```python
from build123d import *

# Parameters (mm, degrees)
F2_DEPTH = 6
F1_W     = 24.3
F1_H     = 10.5
F1_R     = 2.5
F1_W_2   = 4.5
F1_H_2   = 3.75
F1_R_2   = 1.5
F1_R_3   = 20
F3_DEPTH = 6.001
F4_R     = 1
F5_R     = 0.5
F6_R     = 4
F7_R     = 5
F8_R     = 10


# Not quite as in the source:
# - a feature names something its author has since deleted; it is built from what else it names


with BuildPart() as f2:
    # F0 (on Top) → F2 (new body)
    with BuildSketch(Plane.XY):
        with BuildLine():
            Line((-38.5, 52.75), (-38.5, 41.5))
            Line((-38.5, 41.5), (-38.5, -23.99190475))
            ThreePointArc((-38.5, -23.99190475), (-34.7157474887, -63.5877422109), (-23.5, -101.75))
            Line((-23.5, -101.75), (23.5, -101.75))
            ThreePointArc((23.5, -101.75), (34.7157474887, -63.5877422109), (38.5, -23.99190475))
            Line((38.5, -23.99190475), (38.5, 41.5))
            Line((38.5, 41.5), (38.5, 52.75))
            Line((38.5, 52.75), (-38.5, 52.75))
        make_face()
    extrude(amount=F2_DEPTH)

    # F1 (on Top) → F3 (cut, through all)
    with BuildSketch(Plane.XY):
        with Locations((0, -41.5)):
            Rectangle(F1_W, F1_H)
        with BuildLine():
            ThreePointArc((-2.25, -33.25), (-3, -34), (-2.25, -34.75))
            Line((-2.25, -34.75), (2.25, -34.75))
            ThreePointArc((2.25, -34.75), (3, -34), (2.25, -33.25))
            Line((2.25, -33.25), (-2.25, -33.25))
        make_face()
        with BuildLine():
            ThreePointArc((-21, -21.25), (-18.4168483179, -27.5611508459), (-12.15, -30.25))
            Line((-12.15, -30.25), (12.15, -30.25))
            ThreePointArc((12.15, -30.25), (18.4168483179, -27.5611508459), (21, -21.25))
            ThreePointArc((21, -21.25), (25.387505004, -8.75), (21, 3.75))
            Line((21, 3.75), (-21, 3.75))
            ThreePointArc((-21, 3.75), (-25.387505004, -8.75), (-21, -21.25))
        make_face()
        with Locations((-30, 7.75)):
            Circle(F1_R)
        with Locations((-30, 27.75)):
            Circle(F1_R)
        with Locations((30, 7.75)):
            Circle(F1_R)
        with Locations((30, 27.75)):
            Circle(F1_R)
        with Locations((20.35, 41.5)):
            Rectangle(F1_W, F1_H)
        with BuildLine():
            ThreePointArc((18.1, 34.75), (17.35, 34), (18.1, 33.25))
            Line((18.1, 33.25), (22.6, 33.25))
            ThreePointArc((22.6, 33.25), (23.35, 34), (22.6, 34.75))
            Line((22.6, 34.75), (18.1, 34.75))
        make_face()
        with BuildLine():
            ThreePointArc((-22.6, 34.75), (-23.35, 34), (-22.6, 33.25))
            Line((-22.6, 33.25), (-18.1, 33.25))
            ThreePointArc((-18.1, 33.25), (-17.35, 34), (-18.1, 34.75))
            Line((-18.1, 34.75), (-22.6, 34.75))
        make_face()
        with Locations((-20.35, 41.5)):
            Rectangle(F1_W, F1_H)
        with Locations((-20.35, 50.875)):
            Rectangle(F1_W_2, F1_H_2)
        with Locations((20.35, 50.875)):
            Rectangle(F1_W_2, F1_H_2)
        with Locations((0, 46.75)):
            Circle(F1_R_2)
        with Locations((30, -4.25)):
            Circle(F1_R_2)
        with Locations((-30, -4.25)):
            Circle(F1_R_2)
        with Locations((0, -75.75)):
            Circle(F1_R_3)
        with BuildLine():
            ThreePointArc((-2.25, -48.25), (-3, -49), (-2.25, -49.75))
            Line((-2.25, -49.75), (2.25, -49.75))
            ThreePointArc((2.25, -49.75), (3, -49), (2.25, -48.25))
            Line((2.25, -48.25), (-2.25, -48.25))
        make_face()
        with Locations((16, -59.75)):
            Circle(F1_R_2)
        with Locations((-16, -59.75)):
            Circle(F1_R_2)
        with Locations((16, -91.75)):
            Circle(F1_R_2)
        with Locations((-16, -91.75)):
            Circle(F1_R_2)
    extrude(amount=F3_DEPTH, mode=Mode.SUBTRACT)

    # F4
    f4_edges = [f2.edges().sort_by_distance(p)[0] for p in [
        (12.15, -36.25, 3),
        (-12.15, -36.25, 3),
        (-12.15, -46.75, 3),
        (12.15, -46.75, 3),
        (8.2, 46.75, 3),
        (-32.5, 46.75, 3),
        (-32.5, 36.25, 3),
        (-8.2, 46.75, 3),
        (-8.2, 36.25, 3),
        (32.5, 36.25, 3),
        (8.2, 36.25, 3),
        (32.5, 46.75, 3),
    ]]
    fillet(f4_edges, radius=F4_R)

    # F5
    f5_edges = [f2.edges().sort_by_distance(p)[0] for p in [
        (18.1, 49, 3),
        (22.6, 49, 3),
        (-18.1, 49, 3),
        (-22.6, 49, 3),
        (-22.6, 52.75, 3),
        (-18.1, 52.75, 3),
        (18.1, 52.75, 3),
        (22.6, 52.75, 3),
    ]]
    fillet(f5_edges, radius=F5_R)

    # F6
    f6_edges = [f2.edges().sort_by_distance(p)[0] for p in [
        (-21, 3.75, 3),
        (21, 3.75, 3),
    ]]
    fillet(f6_edges, radius=F6_R)

    # F7
    f7_edges = [f2.edges().sort_by_distance(p)[0] for p in [
        (-23.5, -101.75, 3),
        (23.5, -101.75, 3),
        (-38.5, 52.75, 3),
        (38.5, 52.75, 3),
    ]]
    fillet(f7_edges, radius=F7_R)

    # F8
    f8_edges = [f2.edges().sort_by_distance(p)[0] for p in [
        (-21, -21.25, 3),
        (21, -21.25, 3),
    ]]
    fillet(f8_edges, radius=F8_R)


solid = f2.part
```
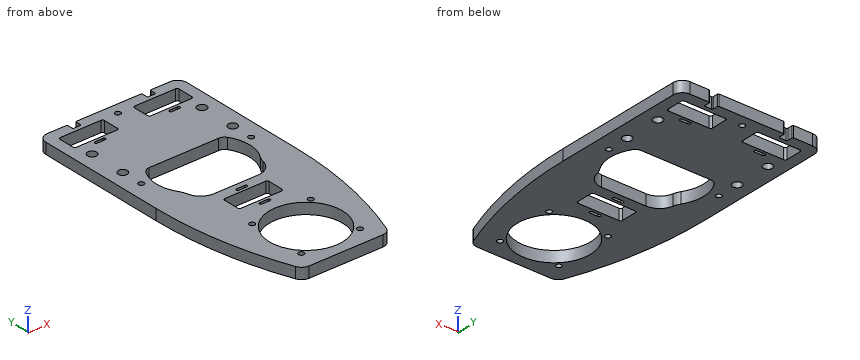
CAD build for the part. Positions are in the model's coordinates, mm. Round coordinates to 2 decimals unless told otherwise and drop trailing zeros. Write each loop counter-clockwise with the first axis right and the second up, starting at its lowest first coordinate (ties: lowest second). Pieces come first, ordered by that corner, then holes. Notation, with made-up numbers: (-18, -9) - (38, -9) arc R35 ccw to (38, 29) - close; hole circle Ø1 at (33.5, -24.5). An arc over 180 degrees is marked (long way). Write item = value, one per line. Start each with the question number.
Q1. Band-saw the part on A-A (x = 0). Give the cut face in (y, z), then the cut area to 3 significant figures.
Q2. Probe L1, parallel to X at y = 7.75, z = 3.15; L2, parallel to Y at x = 7, z = 1 (3 decimals); L3, parallel to Y at x = 4, z = 2.25. List the from-to ranges inside material, lowest first. Write a range as from..to.
Q3. Band-saw the part on C-C (y = -4.25). Give the cut face in (x, z).
Q4. Band-saw the part on D-D (z = 3.25). Count the separate pieces of the cut face and the enclosed holes in it, then the cut area to 3 significant figures.
Q5. Drop flat-ended pins along their axis: pin 1 (0.8 mm diameter, centred on y = 51, z = 3, fed in from +X); pin 2 (4 mm diameter, centred on x = 2.5, y = 28, fed in from -Z); pin 3 (1.3 mm diameter, centred on x = 19.5, z = 2, fed in from +Y); pin 4 (1.4 mm diameter, centred on y = 50.5, z = 1.5, fed in from +X). Give the stop position or say it passes through.
Q6. Band-saw the part on B-B (y = -88). Give the cut face in (x, z).
Answers below:
q1.outline = (-101.75, 0) - (-95.75, 0) - (-95.75, 6) - (-101.75, 6) - close; (-55.75, 0) - (-49.75, 0) - (-49.75, 6) - (-55.75, 6) - close; (-48.25, 0) - (-46.75, 0) - (-46.75, 6) - (-48.25, 6) - close; (-36.25, 0) - (-34.75, 0) - (-34.75, 6) - (-36.25, 6) - close; (-33.25, 0) - (-30.25, 0) - (-30.25, 6) - (-33.25, 6) - close; (3.75, 0) - (45.25, 0) - (45.25, 6) - (3.75, 6) - close; (48.25, 0) - (52.75, 0) - (52.75, 6) - (48.25, 6) - close
q1.area = 384 mm2
q2.L1 = -38.5..-32.5, -27.5..27.5, 32.5..38.5
q2.L2 = -101.75..-94.485, -57.015..-46.75, -36.25..-30.25, 3.75..52.75
q2.L3 = -101.75..-95.35, -56.15..-46.75, -36.25..-30.25, 3.75..52.75
q3.outline = (-38.5, 0) - (-31.5, 0) - (-31.5, 6) - (-38.5, 6) - close; (-28.5, 0) - (-24.87, 0) - (-24.87, 6) - (-28.5, 6) - close; (24.87, 0) - (28.5, 0) - (28.5, 6) - (24.87, 6) - close; (31.5, 0) - (38.5, 0) - (38.5, 6) - (31.5, 6) - close
q4.separate_pieces = 1
q4.enclosed_holes = 20
q4.area = 7,360 mm2
q5.pin_1 = 37.61
q5.pin_2 = 0
q5.pin_3 = 49
q5.pin_4 = 38.06
q6.outline = (-28.46, 0) - (-15.81, 0) - (-15.81, 6) - (-28.46, 6) - close; (15.81, 0) - (28.46, 0) - (28.46, 6) - (15.81, 6) - close
